from build123d import *

# Parameters (mm, degrees)
F_5_8_0_625_DIAMETER_HOLE1_D     = 15.875
F_5_8_0_625_DIAMETER_HOLE1_DEPTH = 69.85
F_5_8_0_625_DIAMETER_HOLE1_TIP   = 4.769331164
CHAMFER1_SIZE                    = 0.635
F_8_32_TAPPED_HOLE1_D            = 3.4544
F_8_32_TAPPED_HOLE1_DEPTH        = 12.7
F_8_32_TAPPED_HOLE1_TIP          = 1.037806461
SKETCH8_R                        = 2.368549992
SKETCH8_R_2                      = 2.368549996
SKETCH8_R_3                      = 2.368550008
SKETCH8_R_4                      = 2.368550004
CUT_EXTRUDE1_DEPTH               = 12.7
CHAMFER2_SIZE                    = 1.524


with BuildPart() as part:
    # Sketch1 → Revolve1 (revolve)
    with BuildSketch(Plane(origin=(0, 0, 0), x_dir=(0, 0, -1), z_dir=(1, 0, 0))):
        Polygon((12.500000019, 108.43719994), (11.949999976, 108.43719994), (11.949999976, 107.1372), (12.500000019, 107.1372), (12.500000019, 0), (6.35, 0), (6.35, 110.97719994), (12.500000019, 110.97719994), align=None)
    revolve(axis=Axis((0, 0, 0), (0, 1, 0)))

    # 5/8 (0.625) Diameter Hole1
    with Locations(Plane(origin=(0, 110.97719994, 0), x_dir=(1, 0, 0), z_dir=(0, 1, 0))):
        with Locations((0, 0)):
            Hole(F_5_8_0_625_DIAMETER_HOLE1_D / 2, depth=F_5_8_0_625_DIAMETER_HOLE1_DEPTH)
            with Locations((0, 0, -(F_5_8_0_625_DIAMETER_HOLE1_DEPTH + F_5_8_0_625_DIAMETER_HOLE1_TIP / 2))):  # 118° drill point
                Cone(0, F_5_8_0_625_DIAMETER_HOLE1_D / 2, F_5_8_0_625_DIAMETER_HOLE1_TIP, mode=Mode.SUBTRACT)

    # Chamfer1
    chamfer1_edges = [part.edges().sort_by_distance(p)[0] for p in [
        (0, 110.97719994, 12.500000019),
    ]]
    chamfer(chamfer1_edges, length=CHAMFER1_SIZE)

    # #8-32 Tapped Hole1
    with Locations(Plane(origin=(0, 0, 0), x_dir=(-1, 0, 0), z_dir=(0, -1, 0))):
        with Locations((9.42500001, 0), (0, -9.42500001), (-9.42500001, 0), (0, 9.42500001)):
            Hole(F_8_32_TAPPED_HOLE1_D / 2, depth=F_8_32_TAPPED_HOLE1_DEPTH)
            with Locations((0, 0, -(F_8_32_TAPPED_HOLE1_DEPTH + F_8_32_TAPPED_HOLE1_TIP / 2))):  # 118° drill point
                Cone(0, F_8_32_TAPPED_HOLE1_D / 2, F_8_32_TAPPED_HOLE1_TIP, mode=Mode.SUBTRACT)

    # Sketch8 → Cut-Extrude1 (cut)
    with BuildSketch(Plane.XZ):
        with Locations(Location((6.664481419, 6.664481419, 0), (0, 0, 270))):
            Circle(SKETCH8_R)
        with Locations(Location((6.664481419, -6.664481419, 0), (0, 0, 270))):
            Circle(SKETCH8_R_2)
        with Locations(Location((-6.664481419, -6.664481419, 0), (0, 0, 270))):
            Circle(SKETCH8_R_3)
        with Locations(Location((-6.664481419, 6.664481419, 0), (0, 0, 270))):
            Circle(SKETCH8_R_4)
    extrude(amount=-CUT_EXTRUDE1_DEPTH, mode=Mode.SUBTRACT)

    # Chamfer2
    chamfer2_edges = [part.edges().sort_by_distance(p)[0] for p in [
        (7.9375, 110.97719994, 0),
    ]]
    chamfer(chamfer2_edges, length=CHAMFER2_SIZE)


solid = part.part
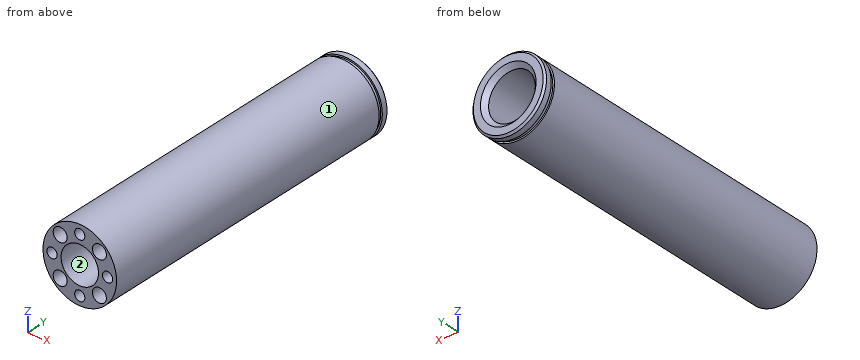
Verification items for the finished model (mm, model axes). Face numbers are marked on the shaded views. Give positions to 0.01 mm unless a question says otherwise; leave off trailing zeros. Loops run counter-clockwise (first coordinate to the right, second up) from the corner with the lowest first, then second, coordinate; pieces in that order, holes last.
1. Go/stop test with flat-tipped pins: P1, Ø2.5, axis at x = 7, z = 5.5, coming from the -Y side; P2, Ø1.4, axis at x = 7, z = -7, coming from the -Y side; P3, Ø1.5, axis at x = 1.5, y = 71, coming from the +Z side; P4, Ø3, axis at x = 0, z = -9.425, coming from the -Y side. Record where each tip stops, or that it passes through.
Derived:
P1: stops at y = 0
P2: stops at y = 12.7
P3: stops at z = 12.48
P4: stops at y = 12.84
2. Cross-section at B-B on y = 46. Record the cut outline in (x, z) (1 decimal), and give its area (3 significant figures).
Derived:
outline: circle Ø25 at (0, 0); hole circle Ø15.9 at (0, 0)
area: 293 mm2
3. Material ranges on probe 1 along Z at (x, y) = (0, 7); probe 2 along X at (y, z) = (95.5, 0), recorded low to high.
Derived:
probe 1: z = -12.5 to -11.15, -7.7 to -6.35, 6.35 to 7.7, 11.15 to 12.5
probe 2: x = -12.5 to -7.94, 7.94 to 12.5
4. Cross-section at A-A on y = 21. Record the cut outline in (x, z), and give its area (3 significant figures).
Derived:
outline: circle Ø25 at (0, 0); hole circle Ø12.7 at (0, 0)
area: 364 mm2
5. Release check for a two-part mould opening along X. For the marked faces 1 and 2 record: +X half, -X half, draft (parallel to the pull), parting line (faces both ways), or undercut.
Derived:
face 1: parting line
face 2: undercut
